Read the model definition and answer for the solid it produces. Units are mm, in the model's axes. Round coordinates to 2 decimals unless told otherwise and drop trailing zeros. Answer as CSV lines item,"result".
```python
from build123d import *

# Parameters (mm, degrees)
EXTRUDE_1_DEPTH     = 4
SKETCH_3_R          = 1.5
CUT_EXTRUDE_1_DEPTH = 184.032783949


with BuildPart() as part:
    # 草图1 → 凸台-拉伸1 (new body)
    with BuildSketch(Plane(origin=(0, 0, 0), x_dir=(1, 0, 0), z_dir=(0, 1, 0))):
        with BuildLine():
            Line((-119.819061856, 72.980279065), (-162.812846416, 32.966261751))
            ThreePointArc((-162.812846416, 32.966261751), (-165.168654868, 29.638038623), (-166, 25.646075708))
            Line((-166, 25.646075708), (-166, -25.646075708))
            ThreePointArc((-166, -25.646075708), (-165.168654868, -29.638038623), (-162.812846416, -32.966261751))
            Line((-162.812846416, -32.966261751), (-119.819061856, -72.980279065))
            ThreePointArc((-119.819061856, -72.980279065), (-115.090503207, -75.958943119), (-109.599792231, -77))
            Line((-109.599792231, -77), (109.599792231, -77))
            ThreePointArc((109.599792231, -77), (115.090503207, -75.958943119), (119.819061856, -72.980279065))
            Line((119.819061856, -72.980279065), (162.812846416, -32.966261751))
            ThreePointArc((162.812846416, -32.966261751), (165.168654868, -29.638038623), (166, -25.646075708))
            Line((166, -25.646075708), (166, 25.646075708))
            ThreePointArc((166, 25.646075708), (165.168654868, 29.638038623), (162.812846416, 32.966261751))
            Line((162.812846416, 32.966261751), (119.819061856, 72.980279065))
            ThreePointArc((119.819061856, 72.980279065), (115.090503207, 75.958943119), (109.599792231, 77))
            Line((109.599792231, 77), (-109.599792231, 77))
            ThreePointArc((-109.599792231, 77), (-115.090503207, 75.958943119), (-119.819061856, 72.980279065))
        make_face()
    extrude(amount=EXTRUDE_1_DEPTH)

    # 草图3 → 切除-拉伸1 (cut, through all)
    with BuildSketch(Plane(origin=(0, 4, 0), x_dir=(1, 0, 0), z_dir=(0, 1, 0))):
        with Locations(Location((10, -72, 0), (0, 0, 270))):
            Circle(SKETCH_3_R)
        with Locations(Location((0, -72, 0), (0, 0, 270))):
            Circle(SKETCH_3_R)
        with Locations(Location((-10, -72, 0), (0, 0, 270))):
            Circle(SKETCH_3_R)
        with Locations(Location((10, -15, 0), (0, 0, 270))):
            Circle(SKETCH_3_R)
        with Locations(Location((0, -15, 0), (0, 0, 270))):
            Circle(SKETCH_3_R)
        with Locations(Location((-10, -15, 0), (0, 0, 270))):
            Circle(SKETCH_3_R)
        with Locations(Location((10, 15, 0), (0, 0, 270))):
            Circle(SKETCH_3_R)
        with Locations(Location((0, 15, 0), (0, 0, 270))):
            Circle(SKETCH_3_R)
        with Locations(Location((-10, 15, 0), (0, 0, 270))):
            Circle(SKETCH_3_R)
        with Locations(Location((10, 72, 0), (0, 0, 270))):
            Circle(SKETCH_3_R)
        with Locations(Location((0, 72, 0), (0, 0, 270))):
            Circle(SKETCH_3_R)
        with Locations(Location((-10, 72, 0), (0, 0, 270))):
            Circle(SKETCH_3_R)
        with Locations(Location((-100.7, 15, 0), (0, 0, 270))):
            Circle(SKETCH_3_R)
        with Locations(Location((-110.7, 15, 0), (0, 0, 270))):
            Circle(SKETCH_3_R)
        with Locations(Location((-100.7, -15, 0), (0, 0, 270))):
            Circle(SKETCH_3_R)
        with Locations(Location((-110.7, -15, 0), (0, 0, 270))):
            Circle(SKETCH_3_R)
        with Locations(Location((100.7, 15, 0), (0, 0, 270))):
            Circle(SKETCH_3_R)
        with Locations(Location((110.7, 15, 0), (0, 0, 270))):
            Circle(SKETCH_3_R)
        with Locations(Location((100.7, -15, 0), (0, 0, 270))):
            Circle(SKETCH_3_R)
        with Locations(Location((110.7, -15, 0), (0, 0, 270))):
            Circle(SKETCH_3_R)
    extrude(amount=-CUT_EXTRUDE_1_DEPTH, mode=Mode.SUBTRACT)


solid = part.part
```
1) Find section A-A, the plane y = 0.8. Count the separate pieces of the cut face and the enclosed holes in it, then the cut area to 3 significant figures.
Evaluation:
separate pieces,"1"
enclosed holes,"20"
area,"46,200 mm^2"
2) Straight lines are drawn through the part: line 1 (Z direction, x = 111.5, y = 0.2); line 2 (X direction, y = 1.1, z = -72); line 3 (X direction, y = 2, z = 26). For each, find the intervals that lie inside material, in ascending order.
Evaluation:
line 1,"z = -76.88 to -16.27, -13.73 to 13.73, 16.27 to 76.88"
line 2,"x = -120.87 to -11.5, -8.5 to -1.5, 1.5 to 8.5, 11.5 to 120.87"
line 3,"x = -165.99 to 165.99"
3) Determine the mould class of faces 1 (the flat face through (141.62, 1.97, -52.69)), 2 (the flat face through (-141.62, 1.97, 52.69)), 3 (the flat face through (-2, 4, -1)) for opening direction Z: released by +Z, released by -Z, zero draft, split by the parting line, or undercut.
Evaluation:
face 1,"released by -Z"
face 2,"released by +Z"
face 3,"zero draft"
4) This flat-tipped pin is pushed along its axis until it touches: P1, Ø1.8, axis at x = 10, z = -72, coming from the +Y side. Where does it stop, or does it pass through?
Evaluation:
P1,"passes through"
